Could you check a few things on this model? Use its own coordinates, in mm. A direction names the side the tool comes from. Coordinates: 2 decimals unless noted, no trailing zeros. Order: outer loops, then holes, each group sorted by start corner. A loop starts at its lowest first (then second) coordinate and runs counter-clockwise, first axis right, second up. Notation, with made-up numbers: M -23,31 L 15,31 A15 ccw 15,51 Z; hole C 79.25,54.5 d11. An arc over 180 degrees is marked long. Write item = value, one per line. Start each with the question number.
from build123d import *

# Parameters (mm, degrees)
PAD048_DEPTH    = 18
SKETCH114_W     = 32
SKETCH114_H     = 2
POCKET042_DEPTH = 10
SKETCH158_W     = 5
SKETCH158_H     = 5
SKETCH158_W_2   = 3
SKETCH158_H_2   = 6
POCKET062_DEPTH = 8


with BuildPart() as part:
    # Sketch085 → Pad048 (new body)
    with BuildSketch(Plane.XY):
        with BuildLine():
            ThreePointArc((36, 0), (18, 18), (0, 0))
            Line((0, 0), (0, -22))
            Line((36, -22), (0, -22))
            Line((36, -22), (36, 0))
        make_face()
        with BuildLine():
            ThreePointArc((34, 0), (18, 16), (2, 0))
            Line((2, -20), (2, 0))
            Line((2, -20), (34, -20))
            Line((34, 0), (34, -20))
        make_face(mode=Mode.SUBTRACT)
    extrude(amount=PAD048_DEPTH)

    # Sketch114 (on Face10 of Pad048) → Pocket042 (cut)
    with BuildSketch(Plane.XY.offset(18)):
        with Locations((18, -21)):
            Rectangle(SKETCH114_W, SKETCH114_H)
    extrude(amount=-POCKET042_DEPTH, mode=Mode.SUBTRACT)

    # Sketch158 (on Face5 of Pocket042) → Pocket062 (cut)
    with BuildSketch(Plane.XY.offset(18)):
        with Locations((18, 16.678012)):
            Rectangle(SKETCH158_W, SKETCH158_H)
        with Locations((1.5, 0)):
            Rectangle(SKETCH158_W_2, SKETCH158_H_2)
        with Locations((34.5, 0)):
            Rectangle(SKETCH158_W_2, SKETCH158_H_2)
    extrude(amount=-POCKET062_DEPTH, mode=Mode.SUBTRACT)


solid = part.part
(1) Please list where these lines run through material, in increasing order: probe 1 along X at (y, z) = (-12.5, 13.25); probe 2 along Y at (x, z) = (31.5, 2.5); probe 3 along X at (y, z) = (11, 13.5). Write a range as from..to.
(2) Imagine slicing it at A-A on y = -6.5. List the corners of the cut face in (x, z) for me, plus the area to 3 significant figures.
(3) Thinking about a two-plate mould opening in X: for faces 1 (the flat face through (36, -11, 9)), 2 (the flat face through (1, -12, 18)), 3 (the flat face through (2, -11, 9)), which applies, released by +X, released by -X, zero draft, split by the parting line, or undercut?
(4) For faces 4 (the flat face through (18, -21, 8)), 5 (the flat face through (1, -3, 14)), 6 (the flat face through (18, -20, 4)), 7 (the flat face through (6, 12, 18)), 8 (the flat face through (20.5, 17, 14)), which set-ups out of +Z, -Z, +X, -X, +Y, -Y let a thin tool reach every point of the face, with its end or its side?
(5) Imagine slicing it at B-B on x = 18. List the corners of the cut face in (y, z) for me.
(6) Will these pins go through, and if not, where does the flat tip stop? P1, Ø1, axis at x = 1.5, z = 13, coming from the +Y side; P2, Ø4, axis at x = 11.5, z = 4, coming from the +Y side; P3, Ø2, axis at y = 17, z = 15, coming from the -X side.
Response:
q1.probe_1 = 0..2, 34..36
q1.probe_2 = -22..-20, 8.59..11.91
q1.probe_3 = 3.75..6.38, 29.62..32.25
q2.outline = M 0,0 L 2,0 L 2,18 L 0,18 Z; M 34,0 L 36,0 L 36,18 L 34,18 Z
q2.area = 72.0 mm2
q3.face_1 = released by +X
q3.face_2 = zero draft
q3.face_3 = undercut
q4.face_4 = +Z, -Y
q4.face_5 = +Z, +X, -X
q4.face_6 = +Z, -Z
q4.face_7 = +Z, +X, -X, +Y, -Y
q4.face_8 = +Z, +Y, -Y
q5.outline = M -22,0 L -20,0 L -20,8 L -22,8 Z; M 16,0 L 18,0 L 18,10 L 16,10 Z
q6.P1 = 8.25
q6.P2 = 17.43
q6.P3 = 9.75
